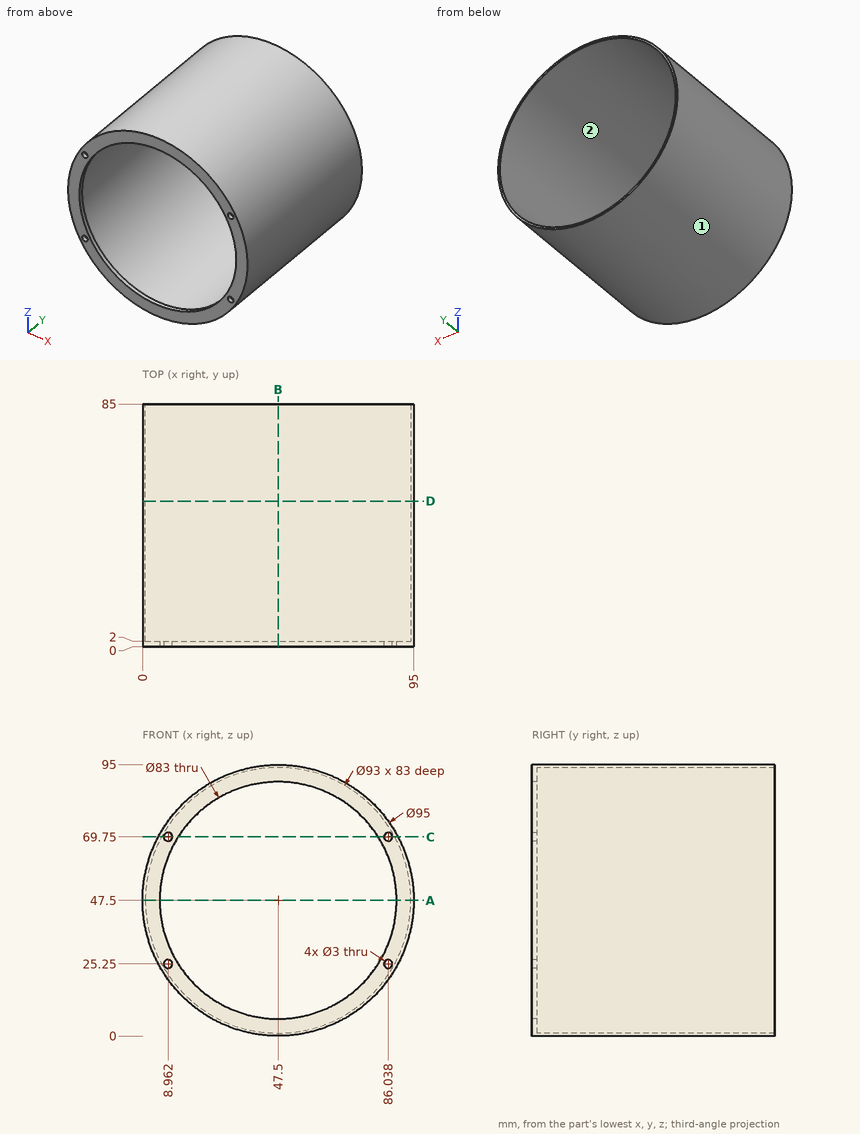
Part print with two shaded views. Sizes in mm from the minimum x, y, z corner. Give positions to 0.01 mm unless a question says otherwise; leave off trailing zeros. Loops run counter-clockwise (first coordinate to the right, second up) from the corner with the lowest first, then second, coordinate; pieces in that order, holes last. Notation, with made-up numbers: (62.5, 35.5) -> (74.5, 35.5) arc R35 ccw to (74.5, 74.5) -> close; hole circle Ø1 at (75.25, 35.5). An arc over 180 degrees is marked (long way). One line per question, with ' | ' between items.
Q1. Cut at A-A, the plane z = 47.5. Write the cut outline in (x, y), plus the area to 3 significant figures.
Filled sheet:
outline: (0, 0) -> (6, 0) -> (6, 2) -> (1, 2) -> (1, 85) -> (0, 85) -> close; (89, 0) -> (95, 0) -> (95, 85) -> (94, 85) -> (94, 2) -> (89, 2) -> close | area: 190 mm²
Q2. Cut at B-B, the plane x = 47.5. Write the cut outline in (y, z).
Filled sheet:
outline: (0, 0) -> (85, 0) -> (85, 1) -> (2, 1) -> (2, 6) -> (0, 6) -> close; (0, 89) -> (2, 89) -> (2, 94) -> (85, 94) -> (85, 95) -> (0, 95) -> close
Q3. Cut at C-C, the plane z = 69.75. Write the cut outline in (x, y).
Filled sheet:
outline: (5.53, 0) -> (7.46, 0) -> (7.46, 2) -> (6.67, 2) -> (6.67, 85) -> (5.53, 85) -> close; (10.46, 0) -> (12.47, 0) -> (12.47, 2) -> (10.46, 2) -> close; (82.53, 0) -> (84.54, 0) -> (84.54, 2) -> (82.53, 2) -> close; (87.54, 0) -> (89.47, 0) -> (89.47, 85) -> (88.33, 85) -> (88.33, 2) -> (87.54, 2) -> close
Q4. Drill centre lines: line 1 along X through (y, z) = (1, 25); line 2 along X through (y, z) = (0.75, 69.75); line 3 along Z through (x, y) = (47.5, 53). Where is each one in solid material? Low to high. Write a range as [from, to].
Filled sheet:
line 1: x = [5.67, 7.48], [10.44, 12.63], [82.37, 84.56], [87.52, 89.33] | line 2: x = [5.53, 7.46], [10.46, 12.47], [82.53, 84.54], [87.54, 89.47] | line 3: z = [0, 1], [94, 95]
Q5. Drop flat-ended pins along their axis: pin 1 (5 mm diameter, centred on x = 41.5, y = 60.5, fed in from -Z); pin 2 (10 mm diameter, centred on x = 43, y = 20, fed in from +Z); pin 3 (1.8 mm diameter, centred on x = 8.96, z = 69.75, fed in from -Y); pin 4 (3 mm diameter, centred on x = 33, y = 26.5, fed in from +Z). Give the stop position or say it passes through.
Filled sheet:
pin 1: stops at z = 0.13 | pin 2: stops at z = 95 | pin 3: passes through | pin 4: stops at z = 93.19
Q6. Cut at D-D, the plane y = 51. Write the cut outline in (x, z).
Filled sheet:
outline: circle Ø95 at (47.5, 47.5); hole circle Ø93 at (47.5, 47.5)
Q7. Pull direction X, two halves, no side cores. Call the marked faces 1 and 2: pulls with the +X half, pulls with the -X half, needs draft (parallel to the pull), parting line crosses it, or undercut.
Filled sheet:
face 1: parting line crosses it | face 2: undercut
